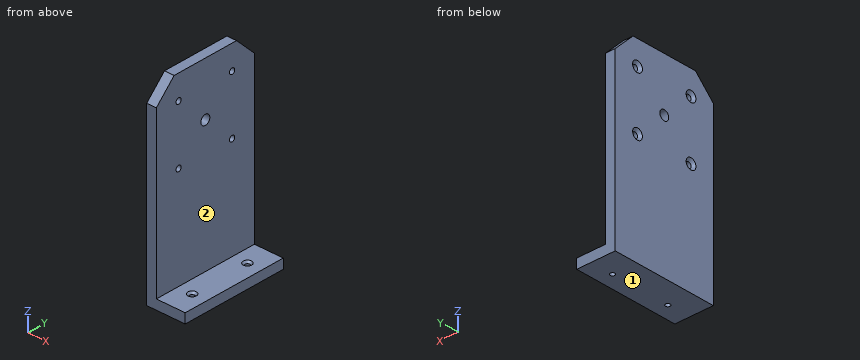
```python
from build123d import *

# Parameters (mm, degrees)
SKETCH1_W                                         = 100
SKETCH1_H                                         = 55
BOSS_EXTRUDE1_DEPTH                               = 5
SKETCH2_W                                         = 5
SKETCH2_H                                         = 55
BOSS_EXTRUDE2_DEPTH                               = 15
CUT_EXTRUDE1_REACH                                = 22
CSK_FOR_M2_FLAT_HEAD_MACHINE_SCREW1_D             = 2.4
CSK_FOR_M2_FLAT_HEAD_MACHINE_SCREW1_CSINK_D       = 4.4
CSK_FOR_M2_FLAT_HEAD_MACHINE_SCREW1_CSINK_ANGLE   = 90
CUT_EXTRUDE2_REACH                                = 22
SKETCH6_R                                         = 2.5
CSK_FOR_M2_5_FLAT_HEAD_MACHINE_SCREW1_D           = 2.9
CSK_FOR_M2_5_FLAT_HEAD_MACHINE_SCREW1_DEPTH       = 5
CSK_FOR_M2_5_FLAT_HEAD_MACHINE_SCREW1_CSINK_D     = 5.5
CSK_FOR_M2_5_FLAT_HEAD_MACHINE_SCREW1_CSINK_ANGLE = 90


with BuildPart() as part:
    # Sketch1 → Boss-Extrude1 (new body)
    with BuildSketch(Plane(origin=(0, 0, 0), x_dir=(0, 0, -1), z_dir=(1, 0, 0))):
        Rectangle(SKETCH1_W, SKETCH1_H)
    extrude(amount=BOSS_EXTRUDE1_DEPTH)

    # Sketch2 → Boss-Extrude2 (add)
    with BuildSketch(Plane(origin=(5, 0, 0), x_dir=(0, 0, -1), z_dir=(1, 0, 0))):
        with Locations((47.5, 0)):
            Rectangle(SKETCH2_W, SKETCH2_H)
    extrude(amount=BOSS_EXTRUDE2_DEPTH)

    # Sketch3 → Cut-Extrude1 (cut, up to next)
    with BuildSketch(Plane.ZY, mode=Mode.PRIVATE) as cut_extrude1_sk1:
        Polygon((50, 27.5), (40, 27.5), (50, 17.5), align=None)
    cut_extrude1_tool1 = extrude(cut_extrude1_sk1.sketch, amount=-CUT_EXTRUDE1_REACH, mode=Mode.PRIVATE) & part.part
    add(cut_extrude1_tool1.solids().sort_by_distance((0, 24.166667, 46.666667))[0], mode=Mode.SUBTRACT)
    # Sketch3 → Cut-Extrude1 (cut, up to next)
    with BuildSketch(Plane.ZY, mode=Mode.PRIVATE) as cut_extrude1_sk2:
        Polygon((50, -27.5), (40, -27.5), (50, -17.5), align=None)
    cut_extrude1_tool2 = extrude(cut_extrude1_sk2.sketch, amount=-CUT_EXTRUDE1_REACH, mode=Mode.PRIVATE) & part.part
    add(cut_extrude1_tool2.solids().sort_by_distance((0, -24.166667, 46.666667))[0], mode=Mode.SUBTRACT)

    # CSK for M2 Flat Head Machine Screw1 (through all)
    with Locations(Plane.XY.offset(-45)):
        with Locations((12.5, 15.5), (12.5, -15.5)):
            CounterSinkHole(CSK_FOR_M2_FLAT_HEAD_MACHINE_SCREW1_D / 2, CSK_FOR_M2_FLAT_HEAD_MACHINE_SCREW1_CSINK_D / 2, counter_sink_angle=CSK_FOR_M2_FLAT_HEAD_MACHINE_SCREW1_CSINK_ANGLE)

    # Sketch6 → Cut-Extrude2 (cut, up to next)
    with BuildSketch(Plane.ZY, mode=Mode.PRIVATE) as cut_extrude2_sk1:
        with Locations((22.5, 0)):
            Circle(SKETCH6_R)
    cut_extrude2_tool1 = extrude(cut_extrude2_sk1.sketch, amount=-CUT_EXTRUDE2_REACH, mode=Mode.PRIVATE) & part.part
    add(cut_extrude2_tool1.solids().sort_by_distance((0, 0, 22.5))[0], mode=Mode.SUBTRACT)

    # CSK for M2.5 Flat Head Machine Screw1
    with Locations(Plane.ZY):
        with Locations((7.5, 15), (7.5, -15), (37.5, -15), (37.5, 15)):
            CounterSinkHole(CSK_FOR_M2_5_FLAT_HEAD_MACHINE_SCREW1_D / 2, CSK_FOR_M2_5_FLAT_HEAD_MACHINE_SCREW1_CSINK_D / 2, depth=CSK_FOR_M2_5_FLAT_HEAD_MACHINE_SCREW1_DEPTH, counter_sink_angle=CSK_FOR_M2_5_FLAT_HEAD_MACHINE_SCREW1_CSINK_ANGLE)


solid = part.part
```
Could you check a few things on this model? Use its own coordinates, in mm. Face numbers are marked on the shaded views. A direction names the side the tool comes from. Round coordinates to 2 decimals unless told otherwise and drop trailing zeros. Loops run counter-clockwise (first coordinate to the right, second up) from the corner with the lowest first, then second, coordinate; pieces in that order, holes last. Notation, with made-up numbers: M 51,55.5 L 87,55.5 A9 ccw 87,60.5 Z; hole C 18.5,14 d3. An arc over 180 degrees is marked long. Answer as CSV lines item,"result".
1) Which directions (+Z, -Z, +X, -X, +Y, -Y) give clear straight access to the entire face, cutting with the end or side of a thin tool? Please do the marked faces 1 and 2.
From the geometry:
face 1,"-Z, +X, -X, +Y, -Y"
face 2,"+Z, +X, +Y, -Y"
2) Imagine slicing it at C-C on y = -23. List the corners of the cut face in (x, z) for me.
From the geometry:
outline,"M 0,-50 L 20,-50 L 20,-45 L 5,-45 L 5,44.5 L 0,44.5 Z"
3) Imagine slicing it at B-B on z = 22.5. List the corners of the cut face in (x, y) for me.
From the geometry:
outline,"M 0,-27.5 L 5,-27.5 L 5,-2.5 L 0,-2.5 Z; M 0,2.5 L 5,2.5 L 5,27.5 L 0,27.5 Z"
4) If I drill on probe 1 along Y at (x, z) = (2.95, 7.5); probe 2 along Y at (x, z) = (12.5, -47.55); probe 3 along Z at (x, y) = (4.25, 15), over which ranges is the centre line in solid material (lowest first)?
From the geometry:
probe 1,"-27.5 to -16.45, -13.55 to 13.55, 16.45 to 27.5"
probe 2,"-27.5 to -16.7, -14.3 to 14.3, 16.7 to 27.5"
probe 3,"-50 to 6.05, 8.95 to 36.05, 38.95 to 50"
5) Imagine slicing it at D-D on y = -1. List the corners of the cut face in (x, z) for me.
From the geometry:
outline,"M 0,-50 L 20,-50 L 20,-45 L 5,-45 L 5,20.21 L 0,20.21 Z; M 0,24.79 L 5,24.79 L 5,50 L 0,50 Z"
6) Imagine slicing it at A-A on x = 12.5. List the corners of the cut face in (y, z) for me.
From the geometry:
outline,"M -27.5,-50 L -16.7,-50 L -16.7,-46 L -17.7,-45 L -27.5,-45 Z; M -14.3,-50 L 14.3,-50 L 14.3,-46 L 13.3,-45 L -13.3,-45 L -14.3,-46 Z; M 16.7,-50 L 27.5,-50 L 27.5,-45 L 17.7,-45 L 16.7,-46 Z"
7) For pin 1 Ø3 at (y, z) = (0, 22.5) entering from +X; pin 2 Ø4.5 at (y, z) = (15, 7.5) entering from -X; pin 3 Ø1.5 at (y, z) = (4, 9.5) entering from -X; pin 4 Ø4 at (y, z) = (14, -5.5) entering from +X, each with a flat end and sliding along its axis, tell me the tip position at first contact or that it passes through.
From the geometry:
pin 1,"through"
pin 2,"x = 0.5"
pin 3,"x = 0"
pin 4,"x = 5"
